from build123d import *

# Parameters (mm, degrees)
SKETCH1_W           = 73.025
SKETCH1_H           = 73.7362
BOSS_EXTRUDE1_DEPTH = 47.6758
SKETCH2_R           = 10.5664
CUT_EXTRUDE1_DEPTH  = 2.54
SKETCH3_R           = 14.732
BOSS_EXTRUDE2_DEPTH = 38.862


with BuildPart() as part:
    # Sketch1 → Boss-Extrude1 (new body)
    with BuildSketch(Plane(origin=(0, 0, 0), x_dir=(1, 0, 0), z_dir=(0, 1, 0))):
        with Locations((36.5125, -36.8681)):
            Rectangle(SKETCH1_W, SKETCH1_H)
    extrude(amount=BOSS_EXTRUDE1_DEPTH)

    # Sketch2 → Cut-Extrude1 (cut)
    with BuildSketch(Plane(origin=(0, 0, 0), x_dir=(-1, 0, 0), z_dir=(0, 0, -1))):
        with Locations((-36.5125, 23.8379)):
            Circle(SKETCH2_R)
    cut_extrude1 = extrude(amount=-CUT_EXTRUDE1_DEPTH, mode=Mode.SUBTRACT)

    # Sketch3 → Boss-Extrude2 (add)
    with BuildSketch(Plane(origin=(0, 47.6758, 0), x_dir=(1, 0, 0), z_dir=(0, 1, 0))):
        with Locations((42.545, -37.465)):
            Circle(SKETCH3_R)
    extrude(amount=BOSS_EXTRUDE2_DEPTH)

    # Mirror1: Cut-Extrude1 across plane
    add(cut_extrude1.mirror(Plane.XY.offset(36.8681)), mode=Mode.SUBTRACT)


solid = part.part
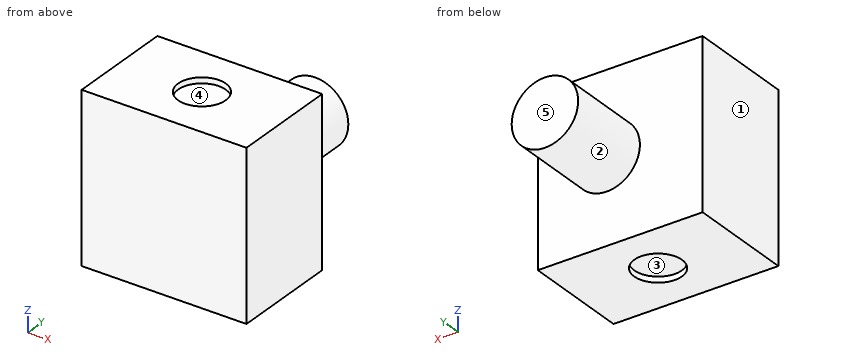
The listing builds one solid part. Answer for the finished solid, in the listing's coordinates (mm). Face numbers are marked on the shaded views. A direction names the side the tool comes from. Round coordinates to 2 decimals unless told otherwise and drop trailing zeros. Write each loop counter-clockwise with the first axis right and the second up, starting at its lowest first coordinate (ties: lowest second). Pieces come first, ordered by that corner, then holes. Notation, with made-up numbers: M -9,76.25 L 9,76.25 A20 ccw 9,115.25 Z; hole C 83.5,20.25 d10. An arc over 180 degrees is marked long. Write each question's results on one line, items separated by ' | '. Start each with the question number.
Item 1: A cutting plane is placed at B-B on z = 56. Write down the section's boundary in (x, y) (3 decimals), and give its area (3 significant figures).
Item 2: A cutting plane is placed at D-D on x = 35. Write down the section's boundary in (y, z).
Item 3: For the marked faces 4 and 5, determine the directions among +Z, -Z, +X, -X, +Y, -Y from which every point of the face is accessible in a straight line to the end or side of a thin tool.
Item 4: A cutting plane is placed at A-A on x = 50.5. Write down the section's boundary in (y, z).
Item 5: For a pull along X with two mould halves and no side action, classify the marked faces 1, 2 and 3 as pulls with the +X half, pulls with the -X half, needs draft (parallel to the pull), parting line crosses it, or undercut.
Item 6: Straight lines are drawn through the part: L1, parallel to Z at x = 30, y = 20; L2, parallel to Y at x = 60.5, z = 29; L3, parallel to X at y = 79.5, z = 33.5. For each, find the intervals that lie inside material, in ascending order. Write a range as [from, to].
Item 7: Flat-ended cylindrical pins translate along their axes: pin 1 Ø6.5 at (x, y) = (39.5, 23.5) entering from +Z; pin 2 Ø8 at (x, y) = (27.5, 57) entering from +Z; pin 3 Ø6.5 at (x, y) = (38, 21) entering from -Z. Find the tip coordinate at first contact, or state that the pin passes through.
Item 8: A cutting plane is placed at C-C on y = 29. Write down the section's boundary in (x, z) (3 decimals).
Check sheet entries:
1) outline: M 0,0 L 73.025,0 L 73.025,47.676 L 0,47.676 Z | area: 3,480 mm²
2) outline: M 0,0 L 13.38,0 L 13.38,2.54 L 34.3,2.54 L 34.3,0 L 47.68,0 L 47.68,24.81 L 86.54,24.81 L 86.54,50.12 L 47.68,50.12 L 47.68,73.74 L 34.3,73.74 L 34.3,71.2 L 13.38,71.2 L 13.38,73.74 L 0,73.74 Z
3) face 4: +Z | face 5: +Z, -Z, +X, -X, +Y
4) outline: M 0,0 L 47.68,0 L 47.68,25.07 L 86.54,25.07 L 86.54,49.86 L 47.68,49.86 L 47.68,73.74 L 0,73.74 Z
5) face 1: pulls with the -X half | face 2: parting line crosses it | face 3: undercut
6) L1: [2.54, 71.2] | L2: [0, 47.68] | L3: [28.36, 56.73]
7) pin 1: z = 71.2 | pin 2: z = 47.21 | pin 3: z = 2.54
8) outline: M 0,0 L 27.293,0 L 27.293,2.54 L 45.732,2.54 L 45.732,0 L 73.025,0 L 73.025,73.736 L 45.732,73.736 L 45.732,71.196 L 27.293,71.196 L 27.293,73.736 L 0,73.736 Z
